from build123d import *

# Parameters (mm, degrees)
SKETCH057_W         = 48
SKETCH057_H         = 56
PAD015_DEPTH        = 2
SKETCH058_R         = 1.75
HOLE023_DEPTH       = 25
SKETCH059_W         = 48
SKETCH059_H         = 32
PAD016_DEPTH        = 30
SKETCH060_W         = 40.4
SKETCH060_H         = 24.4
POCKET018_DEPTH     = 30
SKETCH061_W         = 20
SKETCH061_H         = 20
SKETCH061_W_2       = 40
POCKET019_DEPTH     = 28
SKETCH062_W         = 24
SKETCH062_H         = 22
POCKET020_DEPTH     = 50
SKETCH063_R         = 1.75
HOLE024_DEPTH       = 25
HOLE025_D           = 3.5
HOLE025_DEPTH       = 25
HOLE025_CSINK_D     = 8
HOLE025_CSINK_ANGLE = 90
HOLE025_TIPS_R      = 1.75
FILLET022_R         = 1
FILLET023_R         = 1


with BuildPart() as part:
    # Sketch057 → Pad015 (new body)
    with BuildSketch(Plane.XY):
        Rectangle(SKETCH057_W, SKETCH057_H)
    extrude(amount=PAD015_DEPTH)

    # Sketch058 (on Face6 of Pad015) → Hole023 (cut)
    with BuildSketch(Plane.XY.offset(2)):
        with Locations((18, 22)):
            Circle(SKETCH058_R)
        with Locations((18, -22)):
            Circle(SKETCH058_R)
    hole023 = extrude(amount=-HOLE023_DEPTH, mode=Mode.SUBTRACT)

    # Mirrored028: Hole023 across Sketch058 V_Axis
    add(hole023.mirror(Plane(origin=(0, 0, 2), x_dir=(0, 0, 1), z_dir=(1, 0, 0))), mode=Mode.SUBTRACT)

    # Sketch059 (on Face5 of Mirrored028) → Pad016 (join)
    with BuildSketch(Plane.XY.offset(2)):
        Rectangle(SKETCH059_W, SKETCH059_H)
    extrude(amount=PAD016_DEPTH)

    # Sketch060 (on Face12 of Pad016) → Pocket018 (cut)
    with BuildSketch(Plane.XY.offset(32)):
        Rectangle(SKETCH060_W, SKETCH060_H)
    extrude(amount=-POCKET018_DEPTH, mode=Mode.SUBTRACT)

    # Sketch061 (on Face8 of Pocket018) → Pocket019 (cut)
    with BuildSketch(Plane.XY.offset(32)):
        with Locations((0, 10)):
            Rectangle(SKETCH061_W, SKETCH061_H)
        with Locations((20, 0)):
            Rectangle(SKETCH061_W_2, SKETCH061_H)
    extrude(amount=-POCKET019_DEPTH, mode=Mode.SUBTRACT)

    # Sketch062 (on Face3 of Pocket019) → Pocket020 (cut)
    with BuildSketch(Plane(origin=(-24, 0, 0), x_dir=(0, -1, 0), z_dir=(-1, 0, 0))):
        with Locations((0, 14)):
            Rectangle(SKETCH062_W, SKETCH062_H)
    extrude(amount=-POCKET020_DEPTH, mode=Mode.SUBTRACT)

    # Sketch063 (on Face34 of Pocket020) → Hole024 (cut)
    with BuildSketch(Plane.XY.offset(2)):
        with Locations((-16.2, 8.2)):
            Circle(SKETCH063_R)
        with Locations((-16.2, -8.2)):
            Circle(SKETCH063_R)
    extrude(amount=-HOLE024_DEPTH, mode=Mode.SUBTRACT)

    # Hole025
    with Locations(Plane(origin=(0, 0, 0), x_dir=(1, 0, 0), z_dir=(0, 0, -1))):
        with Locations((-16.2, -8.2), (-16.2, 8.2)):
            CounterSinkHole(HOLE025_D / 2, HOLE025_CSINK_D / 2, depth=HOLE025_DEPTH, counter_sink_angle=HOLE025_CSINK_ANGLE)

    # Hole025 tips → Hole025 tip 1 section 0
    with BuildSketch(Plane(origin=(0, 0, 25), x_dir=(1, 0, 0), z_dir=(0, 0, -1)), mode=Mode.PRIVATE) as hole025_tip_1_s0:
        with Locations((-16.2, -8.2)):
            Circle(HOLE025_TIPS_R)
    loft([hole025_tip_1_s0.sketch, Vertex(-16.2, 8.2, 26.051506)], mode=Mode.SUBTRACT)

    # Hole025 tips → Hole025 tip 2 section 0
    with BuildSketch(Plane(origin=(0, 0, 25), x_dir=(1, 0, 0), z_dir=(0, 0, -1)), mode=Mode.PRIVATE) as hole025_tip_2_s0:
        with Locations((-16.2, 8.2)):
            Circle(HOLE025_TIPS_R)
    loft([hole025_tip_2_s0.sketch, Vertex(-16.2, -8.2, 26.051506)], mode=Mode.SUBTRACT)

    # Fillet022
    fillet022_edges = [part.edges().sort_by_distance(p)[0] for p in [
        (24, -28, 1),
        (24, 28, 1),
        (-24, -28, 1),
        (-24, 28, 1),
    ]]
    fillet(fillet022_edges, radius=FILLET022_R)

    # Fillet023
    fillet023_edges = [part.edges().sort_by_distance(p)[0] for p in [
        (24, 16, 17),
        (-24, 16, 17),
        (24, -16, 17),
        (-24, -16, 17),
    ]]
    fillet(fillet023_edges, radius=FILLET023_R)


solid = part.part
Can you work these out from the model? Positions are in its coordinate system, mm. A direction names the side the tool comes from. Give positions to 0.01 mm unless a question says otherwise; leave off trailing zeros. Loops run counter-clockwise (first coordinate to the right, second up) from the corner with the lowest first, then second, coordinate; pieces in that order, holes last. Notation, with made-up numbers: M 87.25,-25.75 L 138.25,-25.75 A24 cw 138.25,11.25 Z; hole C 5,50 d6. An arc over 180 degrees is marked long. One line per item, written item: value.
1) Thinking about a two-plate mould opening in Y: for faces 4 (the face through (22, -10, 29)), 5 (the face through (0, 14, 4)), 6 (the face through (-22, -12, 14)), which applies, +Y half, -Y half, draft (parallel to the pull), parting line (faces both ways), or undercut?
Geometry check:
face 4: undercut
face 5: draft
face 6: undercut
2) Imagine slicing it at C-C on z = 15. Write out the boundary of the cut face in (x, y).
Geometry check:
outline: M -24,-15 A1 ccw -23,-16 L 23,-16 A1 ccw 24,-15 L 24,-12 L 20.2,-12 L 20.2,-12.2 L -20.2,-12.2 L -20.2,-12 L -24,-12 Z; M -24,12 L -20.2,12 L -20.2,12.2 L -10,12.2 L -10,16 L -23,16 A1 ccw -24,15 Z; M 10,12.2 L 20.2,12.2 L 20.2,12 L 24,12 L 24,15 A1 ccw 23,16 L 10,16 Z
3) Please list where these lines run through material, in increasing order: line 1 (Y direction, x = 18, z = 1); line 2 (Y direction, x = -15, z = 4); line 3 (X direction, y = 12.5, z = 6).
Geometry check:
line 1: y = -28 to -23.75, -20.25 to 20.25, 23.75 to 28
line 2: y = -16 to -12.2, 12.2 to 16
line 3: x = -24 to -10, 10 to 24
4) I'm going to push flat-ended pins straight in: pin 1 (4 mm diameter, centred on x = 21.5, y = 4, fed in from +Z); pin 2 (5.5 mm diameter, centred on x = 18, y = 22, fed in from +Z); pin 3 (3 mm diameter, centred on x = -18, y = 22, fed in from -Z); pin 4 (10 mm diameter, centred on x = -18, z = 9, fed in from +Y). Where does each tip first touch, or does it pass through?
Geometry check:
pin 1: stops at z = 3
pin 2: stops at z = 2
pin 3: passes through
pin 4: stops at y = 16
5) Imagine slicing it at D-D on y = 22. Write out the boundary of the cut face in (x, z).
Geometry check:
outline: M -24,0 L -19.75,0 L -19.75,2 L -24,2 Z; M -16.25,0 L 16.25,0 L 16.25,2 L -16.25,2 Z; M 19.75,0 L 24,0 L 24,2 L 19.75,2 Z
6) On a 3-axis mill with a long thin cutter (end or side, diameter ignored), from which of +Z, -Z, +X, -X, +Y, -Y can I reach the whole of each face in a straight line? I mean faces 1 (the face through (10, 14, 18)), 2 (the face through (22, -11, 25)), 3 (the face through (-14, 12.2, 17)). Say none if no direction works.
Geometry check:
face 1: +Z, +Y
face 2: +X, -X
face 3: +Z
7) Imagine slicing it at B-B on x = 18. Write out the boundary of the cut face in (y, z).
Geometry check:
outline: M -28,0 L -23.75,0 L -23.75,2 L -28,2 Z; M -20.25,0 L 20.25,0 L 20.25,2 L 16,2 L 16,32 L 12.2,32 L 12.2,2 L -12.2,2 L -12.2,32 L -16,32 L -16,2 L -20.25,2 Z; M 23.75,0 L 28,0 L 28,2 L 23.75,2 Z
8) Imagine slicing it at A-A on y = 8.2. Write out the boundary of the cut face in (x, z).
Geometry check:
outline: M -24,0 L -20.2,0 L -18.2,2 L -20.2,2 L -20.2,3 L -24,3 Z; M -24,25 L -20.2,25 L -20.2,32 L -24,32 Z; M -14.2,2 L -12.2,0 L 24,0 L 24,3 L 20.2,3 L 20.2,2 Z
